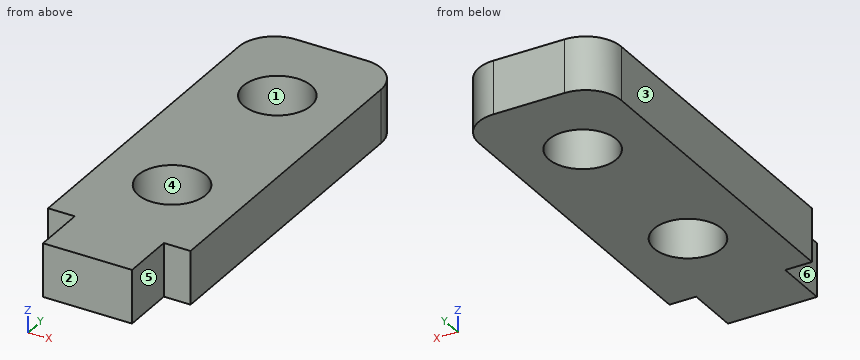
from build123d import *

# Parameters (mm, degrees)
SKETCH1_W             = 8
SKETCH1_H             = 20
SKETCH1_W_2           = 5
SKETCH1_H_2           = 3
BOSS_EXTRUDE1_DEPTH   = 3
F_6_CLEARANCE_HOLE1_D = 3.7973
FILLET1_R             = 2


with BuildPart() as part:
    # Sketch1 → Boss-Extrude1 (new body)
    with BuildSketch(Plane.XY):
        with Locations((0, 13)):
            Rectangle(SKETCH1_W, SKETCH1_H)
        with Locations((0, 1.5)):
            Rectangle(SKETCH1_W_2, SKETCH1_H_2)
    extrude(amount=BOSS_EXTRUDE1_DEPTH)

    # #6 Clearance Hole1 (through all)
    with Locations(Plane.XY.offset(3)):
        with Locations((0, 17.92), (0, 7.98)):
            Hole(F_6_CLEARANCE_HOLE1_D / 2)

    # Fillet1
    fillet1_edges = [part.edges().sort_by_distance(p)[0] for p in [
        (-4, 23, 1.5),
        (4, 23, 1.5),
    ]]
    fillet(fillet1_edges, radius=FILLET1_R)


solid = part.part
Input: part model. Units: mm. Frame: model coordinates. Face numbers are marked on the shaded views. A direction names the side the tool comes from. Coordinates: 2 decimals unless noted, no trailing zeros. Loops run counter-clockwise (first coordinate to the right, second up) from the corner with the lowest first, then second, coordinate; pieces in that order, holes last. Notation, with made-up numbers: (54.25, -30) -> (86.25, -30) arc R7 ccw to (86.25, -25) -> close; hole circle Ø3 at (20.5, 44). An arc over 180 degrees is marked (long way). One line per item, written item: value.
(1) Pin query (flat end, axial travel): pin 1 Ø3 at (x, y) = (0, 17.92) entering from +Z; pin 2 Ø1.6 at (x, z) = (3.5, 2) entering from -Y; pin 3 Ø0.9 at (y, z) = (1, 2) entering from +X. Return the tip coordinate at first contact, or that it passes through.
Answer below:
pin 1: passes through
pin 2: stops at y = 3
pin 3: stops at x = 2.5
(2) Cut plane B-B (z = 2.25). Output: boundary loops of the cut face in (x, y).
Answer below:
outline: (-4, 3) -> (-2.5, 3) -> (-2.5, 0) -> (2.5, 0) -> (2.5, 3) -> (4, 3) -> (4, 21) arc R2 ccw to (2, 23) -> (-2, 23) arc R2 ccw to (-4, 21) -> close; hole circle Ø3.8 at (0, 7.98); hole circle Ø3.8 at (0, 17.92)
(3) Set-up query: the marked faces 4, 5 and 6. Return all of +Z, -Z, +X, -X, +Y, -Y with unobstructed straight access to the full face (end or side cutting, diameter ignored); none if empty.
Answer below:
face 4: +Z, -Z
face 5: +Z, -Z, +X, -Y
face 6: +Z, -Z, -X, -Y
(4) Cut plane C-C (y = 7.98). Output: boundary loops of the cut face in (x, z).
Answer below:
outline: (-4, 0) -> (-1.9, 0) -> (-1.9, 3) -> (-4, 3) -> close; (1.9, 0) -> (4, 0) -> (4, 3) -> (1.9, 3) -> close
(5) Cut plane A-A (x = 0). Output: boundary loops of the cut face in (y, z), then the cut area to 3 significant figures.
Answer below:
outline: (0, 0) -> (6.08, 0) -> (6.08, 3) -> (0, 3) -> close; (9.88, 0) -> (16.02, 0) -> (16.02, 3) -> (9.88, 3) -> close; (19.82, 0) -> (23, 0) -> (23, 3) -> (19.82, 3) -> close
area: 46.2 mm2
(6) Draft query along X for the marked faces 1, 2 and 3. Return one class per face: pulls with the +X half, pulls with the -X half, needs draft (parallel to the pull), parting line crosses it, or undercut.
Answer below:
face 1: undercut
face 2: needs draft
face 3: pulls with the -X half
(7) Ray query, line 1 along Y through (x, z) = (0, 1.6); line 2 along Y through (x, z) = (0.5, 0.4); line 3 along X through (y, z) = (8, 1.55). Return the intervals inside material, ascending.
Answer below:
line 1: y = 0 to 6.08, 9.88 to 16.02, 19.82 to 23
line 2: y = 0 to 6.15, 9.81 to 16.09, 19.75 to 23
line 3: x = -4 to -1.9, 1.9 to 4
(8) Cut plane D-D (y = 2.75). Output: boundary loops of the cut face in (x, z), then the cut area to 3 significant figures.
Answer below:
outline: (-2.5, 0) -> (2.5, 0) -> (2.5, 3) -> (-2.5, 3) -> close
area: 15.0 mm2
